For this review, take the finished solid that the model builds, in its own axes (mm). Face numbers are marked on the shaded views. Round coordinates to 2 decimals unless told otherwise and drop trailing zeros. Loops run counter-clockwise (first coordinate to the right, second up) from the corner with the lowest first, then second, coordinate; pieces in that order, holes last.
1) Take a section at D-D (x = 34). State the section outline as (y, z) points.
2) Mouldability with a two-part tool opening along Y and no side actions: class the marked faces 1, 2 and 3 as pulls with the +Y half, pulls with the -Y half, needs draft (parallel to the pull), parting line crosses it, or undercut.
3) Take a section at A-A (y = -82.55). State the section outline as (x, z) points, then the cut area to 3 significant figures.
4) Take a section at C-C (y = -25.4). State the section outline as (x, z) points, then the cut area to 3 significant figures.
5) Take a section at B-B (x = 25.4). State the section outline as (y, z) points, then the cut area to 3 significant figures.
6) Wall thickness on L1, parallel to Y at x = 25.4, z = 3; L2, parallel to X at y = -82.55, z = 3; L3, parallel to Y at x = 6.35, z = 4.5: over which ranges is each line inside the solid? List them lowest first.
Autodesk Inventor part; units mm, degrees
ref_plane "YZ Plane" through (0, 0, 0) normal (1, 0, 0) x (0, 1, 0)
ref_plane "XZ Plane" through (0, 0, 0) normal (0, 1, 0) x (-1, 0, 0)
ref_plane "XY Plane" through (0, 0, 0) normal (0, 0, 1) x (1, 0, 0)
sketch "Sketch1" plane through (0, 0, 0) normal (0, 0, 1) x (1, 0, 0)
  line L0 (0, 0) -> (50.8, 0)
  line L1 (50.8, 0) -> (50.8, -50.8)
  line L2 (50.8, -50.8) -> (0, -50.8)
  line L3 (0, -50.8) -> (0, 0)
  line L4 (0, -50.8) -> (50.8, -50.8)
  line L5 (50.8, -50.8) -> (50.8, -88.9)
  line L6 (50.8, -88.9) -> (0, -88.9)
  line L7 (0, -88.9) -> (0, -50.8)
  line L8 (0, 0) -> (50.8, -50.8) construction
  circle A0 centre (25.4, -25.4) radius 13.97
  point P0 (42.0116, -42.0116)
  dimension "d0" = 50.8
  dimension "d1" = 50.8
  dimension "d2" = 38.1
  dimension "d3" = 27.94
extrude "Extrusion1" add sketch "Sketch1" along normal blind 6.35
sketch "Sketch2" plane through (0, 0, 6.35) normal (0, 0, 1) x (1, 0, 0)
  circle A0 centre (25.4, -25.4) radius 13.97 construction
  circle A1 centre (25.4, -25.4) radius 25.4 construction
  line L0 (25.4, -25.4) -> (7.4395, -7.4395) construction
  line L1 (25.4, -25.4) -> (50.8, -25.4) construction
  line L2 (25.4, -25.4) -> (43.3605, -43.3605) construction
  line L3 (25.4, -25.4) -> (50.8, -25.4) construction
  point P0 (0, 0)
  dimension "d6" = 50.8
  dimension "d7" = 25.4
  dimension "d8" = 135
  dimension "d9" = 45
hole "Hole1" at (7.4395, -7.4395, 6.35) at (43.3605, -43.3605, 6.35) direction (0, 0, -1) diameter 5.1054 depth 10.795
sketch "Sketch3" plane through (0, 0, 6.35) normal (0, 0, 1) x (1, 0, 0)
  line L0 (0, -88.9) -> (50.8, -88.9) construction
  line L1 (50.8, -88.9) -> (50.8, 0) construction
  line L2 (0, -88.9) -> (50.8, -88.9) construction
  line L3 (50.8, -88.9) -> (50.8, -82.55) construction
  line L4 (50.8, -82.55) -> (0, -82.55) construction
  line L5 (0, -82.55) -> (0, -88.9) construction
  line L6 (0, -82.55) -> (25.4, -82.55) construction
  line L7 (25.4, -82.55) -> (50.8, -82.55) construction
  point P0 (0, 0)
  point P1 (6.35, -82.55)
  point P2 (44.45, -82.55)
  dimension "d17" = 6.35
  dimension "d18" = 19.05
  dimension "d19" = 19.05
hole "Hole2" at (25.4, -82.55, 6.35) at (6.35, -82.55, 6.35) at (44.45, -82.55, 6.35) direction (0, 0, -1) diameter 5.1054 depth 10.795
chamfer "Chamfer1" [suppressed]
properties part number "Versaplanetary Mount"
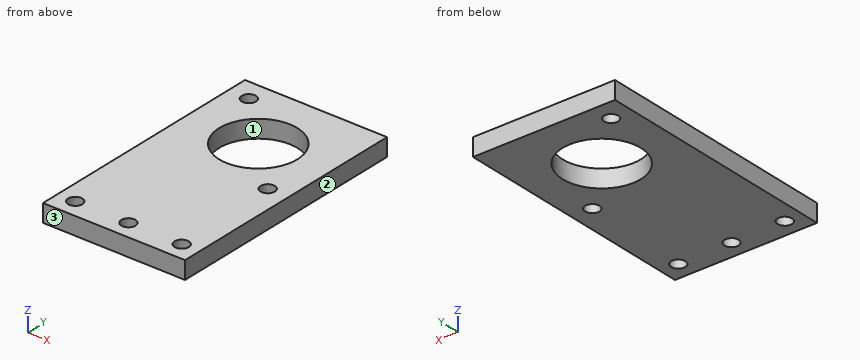
Response:
1. outline: (-88.9, 0) - (-36.41, 0) - (-36.41, 6.35) - (-88.9, 6.35) - close; (-14.39, 0) - (0, 0) - (0, 6.35) - (-14.39, 6.35) - close
2. face 1: undercut
2. face 2: needs draft
2. face 3: pulls with the -Y half
3. outline: (0, 0) - (3.8, 0) - (3.8, 6.35) - (0, 6.35) - close; (8.9, 0) - (22.85, 0) - (22.85, 6.35) - (8.9, 6.35) - close; (27.95, 0) - (41.9, 0) - (41.9, 6.35) - (27.95, 6.35) - close; (47, 0) - (50.8, 0) - (50.8, 6.35) - (47, 6.35) - close
3. area: 225 mm2
4. outline: (0, 0) - (11.43, 0) - (11.43, 6.35) - (0, 6.35) - close; (39.37, 0) - (50.8, 0) - (50.8, 6.35) - (39.37, 6.35) - close
4. area: 145 mm2
5. outline: (-88.9, 0) - (-85.1, 0) - (-85.1, 6.35) - (-88.9, 6.35) - close; (-80, 0) - (-39.37, 0) - (-39.37, 6.35) - (-80, 6.35) - close; (-11.43, 0) - (0, 0) - (0, 6.35) - (-11.43, 6.35) - close
5. area: 355 mm2
6. L1: y = -88.9 to -85.1, -80 to -39.37, -11.43 to 0
6. L2: x = 0 to 3.8, 8.9 to 22.85, 27.95 to 41.9, 47 to 50.8
6. L3: y = -88.9 to -85.1, -80 to -9.75, -5.13 to 0
